from build123d import *

# Parameters (mm, degrees)
F0_W     = 5.919209
F0_H     = 8.541538
F0_R     = 1.251395
F1_DEPTH = 12.7
F2_SIZE  = 5.08


with BuildPart() as f1:
    # F0 (on Front) → F1 (new body, symmetric)
    with BuildSketch(Plane.XZ):
        Polygon((-5.705478, 19.156427), (-21.156731, 19.119902), (-21.156731, 17.007546), (-21.156731, 14.773603), (-17.477301, 14.774974), (-17.477301, 3.613727), (-21.065827, 3.613727), (-21.065827, 0), (-5.71827, 0), (-3.851344, 0), (0, 6.075916), (0, 14.774974), align=None)
        with Locations((-8.607242, 8.278721)):
            Rectangle(F0_W, F0_H, mode=Mode.SUBTRACT)
        with Locations((-17.562349, 16.578252)):
            Circle(F0_R, mode=Mode.SUBTRACT)
        Polygon((6.075916, 0), (0, 6.075916), (-3.851344, 0), (-5.71827, 0), (-5.71827, -2.018174), (-5.71827, -9.968552), (-7.422996, -9.968552), (-7.422996, -13.863573), (1.574568, -13.863573), (1.574568, -10.095728), (0, -10.095728), (0, -3.080508), (6.075916, -8.201027), (12.151833, -3.080508), (12.151833, -10.095728), (10.774577, -10.095728), (10.774577, -13.863573), (19.772141, -13.863573), (19.772141, -10.095728), (17.274087, -10.095728), (17.274087, 1.940169), (19.772141, 1.940169), (19.772141, 6.075916), (12.151833, 6.075916), align=None)
    extrude(amount=F1_DEPTH, both=True)

    # F2
    f2_edges = [f1.edges().sort_by_distance(p)[0] for p in [
        (-5.647637, 0, 4.007952),
    ]]
    chamfer(f2_edges, length=F2_SIZE)


solid = f1.part
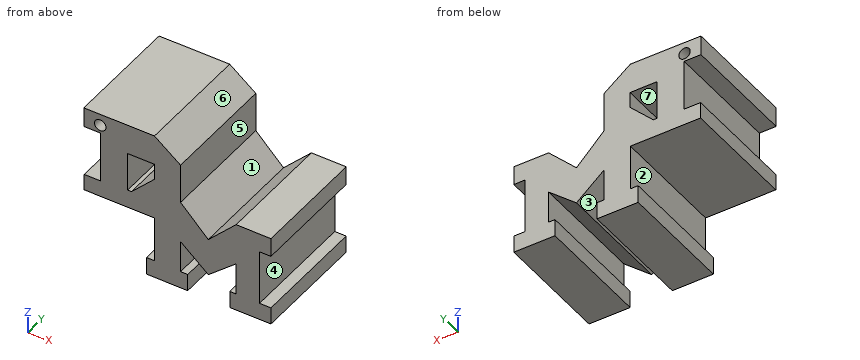
The model under review builds one solid part; all positions refer to its coordinate system, in mm. Face numbers are marked on the shaded views. A direction names the side the tool comes from. Round coordinates to 2 decimals unless told otherwise and drop trailing zeros. Order: outer loops, then holes, each group sorted by start corner. A loop starts at its lowest first (then second) coordinate and runs counter-clockwise, first axis right, second up. Notation, with made-up numbers: (-10.75, 65) -> (-0.75, 65) arc R13 ccw to (-0.75, 90) -> close; hole circle Ø7 at (-29.75, 38). An arc over 180 degrees is marked (long way). Use CSV: the item, a comma, the result in double quotes. Start each with the question number.
(1) Tool access review of the marked faces 1, 2, 3 and 4: name each direction out of +Z, -Z, +X, -X, +Y, -Y from which nothing blocks a thin tool from reaching the whole face with its end or side.
(2) Mouldability with a two-part tool opening along Z and no side actions: class the marked faces 5, 6 and 7 as pulls with the +Z half, pulls with the -Z half, needs draft (parallel to the pull), parting line crosses it, or undercut.
(3) Insertion check: pin 1 (7.5 mm diameter, centred on x = -16.5, y = -1, fed in from -Z); pin 2 (0.5 mm diameter, centred on x = 1, y = -3.5, fed in from +Z); pin 3 (2 mm diameter, centred on x = -14.5, y = 4.5, fed in from +Z). Each pin has a flat end and moves straight along its axis. Give the tip position at first contact, or say it passes through.
(4) Consider section D-D on x = -5. Write out the cut boundary in (y, z), and give its area (3 significant figures).
(5) Consider section C-C on z = -0.5. Write out the cut boundary in (x, y).
(6) Consider section A-A on z = 10. Write out the cut boundary in (x, y).
(7) Consider section B-B on x = 11.5. Write out the cut boundary in (y, z), and give its area (3 significant figures).
(8) Wall thickness on probe 1 along Z at (x, y) = (18.5, -1.5); probe 2 along Z at (x, y) = (16.5, -6.25); probe 3 along X at (y, z) = (8.5, -9): over which ranges is each line inside the solid? List them lowest first. Write a range as from..to.
Responses:
1,face 1,"+Z, +Y, -Y"
1,face 2,"-X, +Y, -Y"
1,face 3,"+Y, -Y"
1,face 4,"+X, +Y, -Y"
2,face 5,"needs draft"
2,face 6,"pulls with the +Z half"
2,face 7,"undercut"
3,pin 1,"z = 0"
3,pin 2,"z = 5.33"
3,pin 3,"z = 19.14"
4,outline,"(-12.7, -13.86) -> (12.7, -13.86) -> (12.7, 18.61) -> (-12.7, 18.61) -> close"
4,area,"825 mm²"
5,outline,"(-5.72, -12.7) -> (17.27, -12.7) -> (17.27, 12.7) -> (-5.72, 12.7) -> close"
6,outline,"(-17.48, -12.7) -> (-11.57, -12.7) -> (-11.57, 12.7) -> (-17.48, 12.7) -> close; (-5.65, -12.7) -> (0, -12.7) -> (0, 12.7) -> (-5.65, 12.7) -> close"
7,outline,"(-12.7, -13.86) -> (12.7, -13.86) -> (12.7, -10.1) -> (-12.7, -10.1) -> close; (-12.7, -3.63) -> (12.7, -3.63) -> (12.7, 5.42) -> (-12.7, 5.42) -> close"
7,area,"326 mm²"
8,probe 1,"-13.86..-10.1, 1.94..6.08"
8,probe 2,"-13.86..6.08"
8,probe 3,"-5.72..0, 12.15..17.27"
